Geometry check sheet. Reference: the model listing, model coordinates, mm. Face numbers are marked on the shaded views. Coordinates: 2 decimals unless noted, no trailing zeros. Write each loop counter-clockwise with the first axis right and the second up, starting at its lowest first coordinate (ties: lowest second). Pieces come first, ordered by that corner, then holes. Notation, with made-up numbers: (74.25, 47.5) -> (127.25, 47.5) arc R12 cw to (127.25, 68.5) -> close; hole circle Ø6 at (59.25, 69). An arc over 180 degrees is marked (long way). Put each result on its own line as item: value. Start each with the question number.
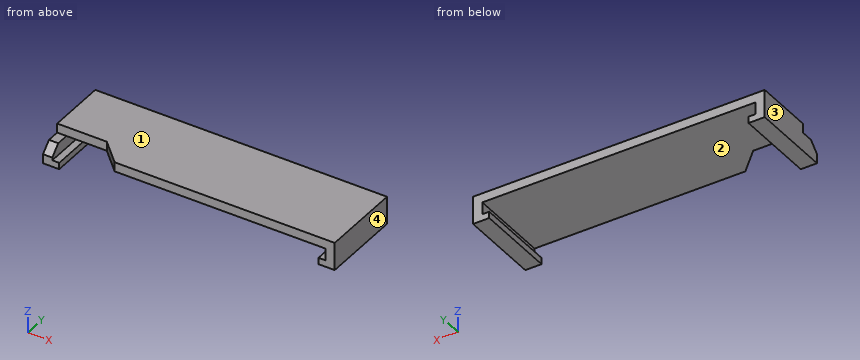
Autodesk Inventor part; units mm, degrees
ref_plane "РабПлоскость1" through (31.45, 0, 2) normal (-1, 0, 0) x (0, 0, 1)
ref_plane "РабПлоскость2" through (0, 4, 2) normal (0, 1, 0) x (1, 0, 0)
ref_plane "YZ Plane" through (0, 0, 0) normal (1, 0, 0) x (0, 1, 0)
sketch "Эскиз1" plane through (0, 0, 0) normal (0, 0, 1) x (1, 0, 0)
  line L0 (0, 0) -> (62.9, 0)
  line L1 (62.9, 0) -> (62.9, 8)
  line L2 (62.9, 8) -> (0, 8)
  line L3 (0, 8) -> (0, 0)
  dimension "d0" = 62.9
  dimension "d1" = 8
extrude "Выдавливание1" add sketch "Эскиз1" along normal blind 2
sketch "Эскиз2" plane through (0, 8, 0) normal (0, 1, 0) x (1, 0, 0)
  line L0 (0, 0) -> (2, 0)
  line L1 (2, 0) -> (2, 4)
  line L2 (2, 4) -> (0, 4)
  line L3 (0, 4) -> (0, 0)
  line L4 (2, 4) -> (3.5, 4)
  line L5 (3.5, 4) -> (3.5, 2.6)
  line L6 (3.5, 2.6) -> (2, 2.6)
  line L7 (2, 2.6) -> (2, 4)
  point P0 (2, 2.6)
  point P1 (2, 2.6)
  dimension "d4" = 2
  dimension "d5" = 4
  dimension "d6" = 1.5
  dimension "d7" = 1.4
extrude "Выдавливание2" add sketch "Эскиз2" against normal up to surface (8 mm away)
ref_plane "РабПлоскость1" through (31.45, 0, 2) normal (-1, 0, 0) x (0, 0, 1)
mirror "Зеркальное отражение1" about plane through (31.45, 0, 2) normal (-1, 0, 0) of "Выдавливание2"
sketch "Эскиз6" plane through (0, 0, 2) normal (0, -1, 0) x (1, 0, 0)
  line L0 (62.9, -2) -> (10.7, -2)
  line L1 (10.7, -2) -> (10.7, 0)
  line L2 (10.7, 0) -> (62.9, 0)
  line L3 (62.9, 0) -> (62.9, -2)
  line L4 (2, -2) -> (60.9, -2)
  line L5 (0, 0) -> (62.9, 0)
  line L6 (2, -2) -> (60.9, -2)
  line L7 (60.9, -2) -> (60.9, -4.6)
  line L8 (60.9, -4.6) -> (59.4, -4.6)
  line L9 (59.4, -4.6) -> (59.4, -6)
  line L10 (59.4, -6) -> (62.9, -6)
  line L11 (62.9, -6) -> (62.9, 0)
  line L12 (0, 0) -> (62.9, 0)
  line L13 (0, -6) -> (0, 0)
  line L14 (3.5, -6) -> (0, -6)
  line L15 (3.5, -4.6) -> (3.5, -6)
  line L16 (2, -4.6) -> (3.5, -4.6)
  line L17 (2, -2) -> (2, -4.6)
  line L18 (60.9, -2) -> (62.9, -2)
  line L19 (2, -2) -> (0, -2)
  line L20 (62.9, -6) -> (62.9, 0)
  point P0 (0, -2)
  dimension "d29" = 10.7
extrude "Выдавливание6" add sketch "Эскиз6" along normal blind 4.75 contours L11 L10 L9 L8 L7 L0 | L0 L1 L2 L3 | L17 L16 L15 L14 L13 L19
ref_plane "РабПлоскость2" through (0, 4, 2) normal (0, 1, 0) x (1, 0, 0)
sketch "Эскиз7" plane through (0, 8, 2) normal (0, 1, 0) x (1, 0, 0)
  line L0 (60.9, 2) -> (2, 2)
  line L1 (2, 2) -> (2, 4.6)
  line L2 (2, 4.6) -> (3.5, 4.6)
  line L3 (3.5, 4.6) -> (3.5, 6)
  line L4 (3.5, 6) -> (0, 6)
  line L5 (0, 6) -> (0, 0)
  line L6 (62.9, 0) -> (0, 0)
  line L7 (62.9, 6) -> (62.9, 0)
  line L8 (59.4, 6) -> (62.9, 6)
  line L9 (59.4, 4.6) -> (59.4, 6)
  line L10 (60.9, 4.6) -> (59.4, 4.6)
  line L11 (60.9, 2) -> (60.9, 4.6)
  point P0 (0, 2)
extrude "Выдавливание7" add sketch "Эскиз7" along normal blind 4.75
sketch "Эскиз5" plane through (0, 0, 2) normal (0, 0, 1) x (1, 0, 0)
  line L0 (49.7, 12.75) -> (47.2, 12.75)
  line L1 (47.2, 12.75) -> (47.2, 4.75)
  line L2 (47.2, 4.75) -> (49.7, 4.75)
  line L3 (49.7, 4.75) -> (49.7, 12.75)
  line L4 (62.9, 0) -> (62.9, 8)
  line L5 (62.9, 4) -> (49.7, 4)
  line L6 (0, 12.75) -> (62.9, 12.75)
  point P0 (0, 0)
  dimension "d15" = 2.5
  dimension "d16" = 8
  dimension "d19" = 13.2
extrude "Выдавливание5" [suppressed]
chamfer "Фаска1" distance 4.75 angle 45 1 edges at (10.7, -4.75, 1)
chamfer "Фаска2" distance 2 angle 45 1 edges at (1, -4.75, 0)
properties part number "Крышка аккумулятора"
Item 1: Section check C-C, the plane x = 6.5. Enter the section's corners in (y, z), and give its area (3 significant figures).
Item 2: Scan lines: line 1 along X through (y, z) = (-1, -0.25); line 2 along Z through (x, y) = (60, 1.25); line 3 along Z through (x, y) = (52, 8.5). Record each from-to range of solid material in increasing order. Write a range as [from, to].
Item 3: Mould release check, pull along X, two halves, no side actions. Record for the marked faces 1, 2, 3 and 4: released by +X, released by -X, zero draft, split by the parting line, or undercut.
Item 4: Section check B-B, the plane y = -1. Enter the section's corners in (x, z).
Item 5: Section check A-A, the plane z = -0.85. Enter the section's corners in (x, y), and give its area (3 significant figures).
Item 6: Section check D-D, the plane y = -3.5. Enter the section's corners in (x, z).
Item 7: Go/stop test with flat-tipped pins: P1, Ø1.5, axis at x = 27, z = -0.5, coming from the +Y side; P2, Ø1, axis at x = 3.5, z = 1, coming from the -Y side; P3, Ø2, axis at x = 1.5, y = -2, coming from the +Z side. Record where each tip stops, or that it passes through.
From the geometry:
1. outline: (0, 0) -> (12.75, 0) -> (12.75, 2) -> (0, 2) -> close
1. area: 25.5 mm²
2. line 1: [0, 2], [60.9, 62.9]
2. line 2: [-4, -2.6], [0, 2]
2. line 3: [0, 2]
3. face 1: zero draft
3. face 2: undercut
3. face 3: released by -X
3. face 4: released by +X
4. outline: (0, -4) -> (3.5, -4) -> (3.5, -2.6) -> (2, -2.6) -> (2, 0) -> (0, 0) -> close; (11.7, 0) -> (60.9, 0) -> (60.9, -2.6) -> (59.4, -2.6) -> (59.4, -4) -> (62.9, -4) -> (62.9, 2) -> (11.7, 2) -> close
5. outline: (0, -3.6) -> (2, -3.6) -> (2, 12.75) -> (0, 12.75) -> close; (60.9, -4.75) -> (62.9, -4.75) -> (62.9, 12.75) -> (60.9, 12.75) -> close
5. area: 67.7 mm²
6. outline: (0, -4) -> (3.5, -4) -> (3.5, -2.6) -> (2, -2.6) -> (2, -0.75) -> (0, -0.75) -> close; (14.2, 0) -> (60.9, 0) -> (60.9, -2.6) -> (59.4, -2.6) -> (59.4, -4) -> (62.9, -4) -> (62.9, 2) -> (14.2, 2) -> close
7. P1: y = 12.75
7. P2: y = 0
7. P3: z = 0
